Can you work these out from the model? Positions are in its coordinate system, mm. Face numbers are marked on the shaded views. Coordinates: 2 decimals unless noted, no trailing zeros. Order: outer loops, then holes, each group sorted by start corner. A loop starts at its lowest first (then second) coordinate and runs counter-clockwise, first axis right, second up.
```python
from build123d import *

# Parameters (mm, degrees)
SKETCH1_W           = 100
SKETCH1_H           = 60
BOSS_EXTRUDE1_DEPTH = 10
SHELL1_T            = -2
FILLET1_R           = 2
SKETCH2_W           = 5
SKETCH2_H           = 1
SKETCH2_W_2         = 10
SKETCH2_H_2         = 3
CUT_EXTRUDE1_DEPTH  = 2


with BuildPart() as part:
    # Sketch1 → Boss-Extrude1 (new body)
    with BuildSketch(Plane(origin=(0, 0, 0), x_dir=(1, 0, 0), z_dir=(0, 1, 0))):
        Rectangle(SKETCH1_W, SKETCH1_H)
    extrude(amount=BOSS_EXTRUDE1_DEPTH)

    # Shell1
    shell1_openings = [part.faces().sort_by_distance(p)[0] for p in [
        (0, 10, 0),
    ]]
    offset(amount=SHELL1_T, openings=shell1_openings, kind=Kind.INTERSECTION)

    # Fillet1
    fillet1_edges = [part.edges().sort_by_distance(p)[0] for p in [
        (0, 0, -30),
        (50, 0, 0),
        (0, 0, 30),
        (-50, 0, 0),
        (-50, 5, -30),
        (50, 5, -30),
        (50, 5, 30),
        (-50, 5, 30),
    ]]
    fillet(fillet1_edges, radius=FILLET1_R)

    # Sketch2 → Cut-Extrude1 (cut)
    with BuildSketch(Plane.ZY.offset(50)):
        with Locations((-6.5, 6)):
            Rectangle(SKETCH2_W, SKETCH2_H)
        with Locations((-18, 6)):
            Rectangle(SKETCH2_W_2, SKETCH2_H_2)
    extrude(amount=-CUT_EXTRUDE1_DEPTH, mode=Mode.SUBTRACT)


solid = part.part
```
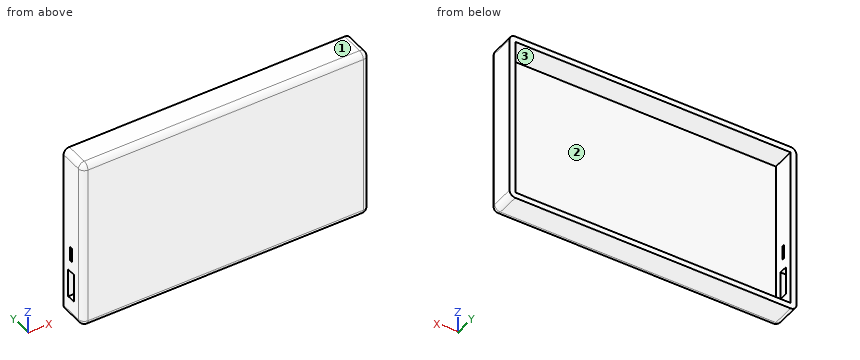
1. Imagine slicing it at A-A on z = -5. Please give me the cut outline in (x, y).
Completed:
outline: (-50, 2) arc R2 ccw to (-48, 0) - (48, 0) arc R2 ccw to (50, 2) - (50, 10) - (48, 10) - (48, 2) - (-48, 2) - (-48, 5.5) - (-50, 5.5) - close; (-50, 6.5) - (-48, 6.5) - (-48, 10) - (-50, 10) - close
2. Thinking about a two-plate mould opening in X: for the marked faces 1, 2 and 3, which applies, pulls with the +X half, pulls with the -X half, needs draft (parallel to the pull), parting line crosses it, or undercut?
Completed:
face 1: needs draft
face 2: undercut
face 3: undercut
3. Imagine slicing it at D-D on z = -16.5. Please give me the cut outline in (x, y), then the cut area to 3 significant figures.
Completed:
outline: (-50, 2) arc R2 ccw to (-48, 0) - (48, 0) arc R2 ccw to (50, 2) - (50, 10) - (48, 10) - (48, 2) - (-48, 2) - (-48, 4.5) - (-50, 4.5) - close; (-50, 7.5) - (-48, 7.5) - (-48, 10) - (-50, 10) - close
area: 224 mm2
4. Please list where these lines run through material, in increasing order: probe 1 along X at (y, z) = (8.5, -6); probe 2 along Z at (x, y) = (-28, 3.75); probe 3 along Y at (x, z) = (-5, -22).
Completed:
probe 1: x = -50 to -48, 48 to 50
probe 2: z = -30 to -28, 28 to 30
probe 3: y = 0 to 2
5. Imagine slicing it at B-B on x = -25. Please give me the cut outline in (y, z).
Completed:
outline: (0, -28) arc R2 ccw to (2, -30) - (10, -30) - (10, -28) - (2, -28) - (2, 28) - (10, 28) - (10, 30) - (2, 30) arc R2 ccw to (0, 28) - close
6. I'm going to push flat-ended pins straight in: pin 1 (1.6 mm diameter, centred on x = -49.5, y = 6, fed in from +Z); pin 2 (10 mm diameter, centred on x = 30, z = 9.5, fed in from +Y); pin 3 (0.6 mm diameter, centred on x = -49, z = -19.5, fed in from -Y). Where does each tip first touch, or does it pass through?
Completed:
pin 1: stops at z = 29.87
pin 2: stops at y = 2
pin 3: stops at y = 0.13
7. Imagine slicing it at C-C on z = 1. Please give me the cut outline in (x, y).
Completed:
outline: (-50, 2) arc R2 ccw to (-48, 0) - (48, 0) arc R2 ccw to (50, 2) - (50, 10) - (48, 10) - (48, 2) - (-48, 2) - (-48, 10) - (-50, 10) - close
